Input: part model. Units: mm. Frame: model coordinates. Face numbers are marked on the shaded views. A direction names the side the tool comes from. Round coordinates to 2 decimals unless told otherwise and drop trailing zeros. Loops run counter-clockwise (first coordinate to the right, second up) from the corner with the lowest first, then second, coordinate; pieces in that order, holes last. Notation, with made-up numbers: M 1.25,31.25 L 36.25,31.25 A15 ccw 36.25,48.25 Z; hole C -37,59 d8. An arc over 180 degrees is marked long. Return JSON: item names as keys, results as strings. Group by question number.
1) Section C-C (z = 12). Output: boundary loops of the cut face in (x, y), plus the area to 3 significant figures.
2) Section B-B (x = 8.5). Output: boundary loops of the cut face in (y, z).
3) Material intervals for line 1 (Z direction, x = -2.5, y = 2); line 2 (Y direction, x = 7, z = 23); line 3 (Y direction, x = 3, z = -13.5), sorted ascending. Write a range as from..to.
4) Section D-D (x = -10.5). Output: boundary loops of the cut face in (y, z).
5) Section A-A (y = 2). Output: boundary loops of the cut face in (x, z).
6) Access query for the marked faces 1 and 2. Directions: +Z, -Z, +X, -X, +Y, -Y. A direction counts if a zero-diameter tool reaches every point of the face in a straight line with its end or side. Return the directions, or none.
7) Contact query for flat-ended pins moving along their axis: P1, Ø1, axis at x = 2, y = 2, coming from the -Z side; P2, Ø11, axis at x = 7, z = 25, coming from the +Y side; P3, Ø1.4, axis at y = 2.5, z = -17, coming from the -X side. Output: stop coordinate, or through.
from build123d import *

# Parameters (mm, degrees)
SKETCH_1_W          = 32.2
SKETCH_1_H          = 49.23
EXTRUDE_1_DEPTH     = 1.2
SKETCH_2_W          = 20.32
SKETCH_2_H          = 2
EXTRUDE_2_DEPTH     = 1.8
SKETCH_2_3_R        = 1.75
CUT_EXTRUDE_1_DEPTH = 1.8
EXTRUDE_3_DEPTH     = 1.46


with BuildPart() as part:
    # Sketch 1 → Extrude 1 (new body)
    with BuildSketch(Plane(origin=(0, 0, 0), x_dir=(1, 0, 0), z_dir=(0, 1, 0))):
        with Locations((0.963198928, -6.298805668)):
            Rectangle(SKETCH_1_W, SKETCH_1_H)
    extrude(amount=EXTRUDE_1_DEPTH)

    # Sketch 2 → Extrude 2 (add)
    with BuildSketch(Plane(origin=(0, 1.2, 0), x_dir=(1, 0, 0), z_dir=(0, 1, 0))):
        with Locations((0.963198928, 16.816194332)):
            Rectangle(SKETCH_2_W, SKETCH_2_H)
    extrude(amount=EXTRUDE_2_DEPTH)

    # Sketch 2_3 → Cut-Extrude 1 (cut)
    with BuildSketch(Plane(origin=(0, 1.2, 0), x_dir=(1, 0, 0), z_dir=(0, 1, 0))):
        with Locations(Location((15.063198928, -28.913805668, 0), (0, 0, 270))):
            Circle(SKETCH_2_3_R)
        with Locations(Location((15.063198928, 16.316194332, 0), (0, 0, 270))):
            Circle(SKETCH_2_3_R)
        with Locations(Location((-13.136801072, 16.316194332, 0), (0, 0, 270))):
            Circle(SKETCH_2_3_R)
        with Locations(Location((-13.136801072, -28.913805668, 0), (0, 0, 270))):
            Circle(SKETCH_2_3_R)
    extrude(amount=-CUT_EXTRUDE_1_DEPTH, mode=Mode.SUBTRACT)

    # Sketch 3 → Extrude 3 (add)
    with BuildSketch(Plane(origin=(0, 1.2, 0), x_dir=(1, 0, 0), z_dir=(0, 1, 0))):
        with BuildLine():
            Line((-9.986801072, 13.316194332), (11.913198928, 13.316194332))
            ThreePointArc((11.913198928, 13.316194332), (15.554798851, 11.807794255), (17.063198928, 8.166194332))
            Line((17.063198928, 8.166194332), (17.063198928, -20.763805668))
            ThreePointArc((17.063198928, -20.763805668), (15.554798851, -24.405405591), (11.913198928, -25.913805668))
            Line((11.913198928, -25.913805668), (-9.986801072, -25.913805668))
            ThreePointArc((-9.986801072, -25.913805668), (-13.628400995, -24.405405591), (-15.136801072, -20.763805668))
            Line((-15.136801072, -20.763805668), (-15.136801072, 8.166194332))
            ThreePointArc((-15.136801072, 8.166194332), (-13.628400995, 11.807794255), (-9.986801072, 13.316194332))
        make_face()
    extrude(amount=EXTRUDE_3_DEPTH)


solid = part.part
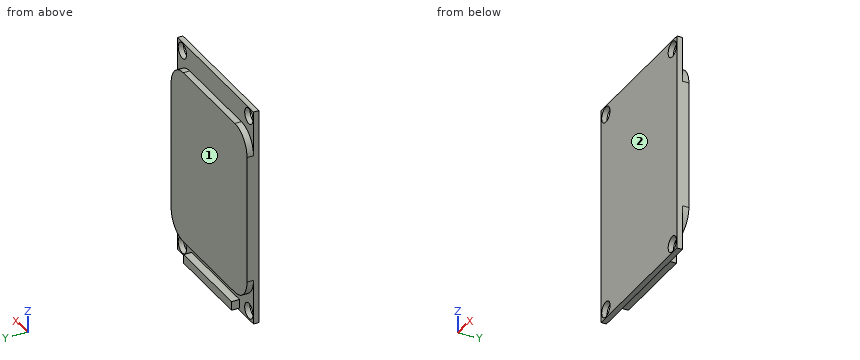
Returned:
{
 "1": {"outline": "M -15.14,0 L 17.06,0 L 17.06,2.66 L -15.14,2.66 Z", "area": "85.7 mm^2"},
 "2": {"outline": "M 0,-18.32 L 1.2,-18.32 L 1.2,-17.82 L 3,-17.82 L 3,-15.82 L 1.2,-15.82 L 1.2,-13.32 L 2.66,-13.32 L 2.66,25.91 L 1.2,25.91 L 1.2,30.91 L 0,30.91 Z"},
 "3": {"line 1": "z = -17.82..-15.82, -13.32..25.91", "line 2": "y = 0..2.66", "line 3": "y = 0..1.2"},
 "4": {"outline": "M 0,-18.32 L 1.2,-18.32 L 1.2,-13.29 L 2.66,-13.29 L 2.66,25.89 L 1.2,25.89 L 1.2,30.91 L 0,30.91 Z"},
 "5": {"outline": "M -15.14,-8.17 A5.15 ccw -9.99,-13.32 L 11.91,-13.32 A5.15 ccw 17.06,-8.17 L 17.06,20.76 A5.15 ccw 11.91,25.91 L -9.99,25.91 A5.15 ccw -15.14,20.76 Z; M -9.2,-17.82 L 11.12,-17.82 L 11.12,-15.82 L -9.2,-15.82 Z"},
 "6": {"face 1": "+Z, +X, -X, +Y", "face 2": "+Z, -Z, +X, -X, -Y"},
 "7": {"P1": "stops at z = -17.82", "P2": "stops at y = 2.66", "P3": "stops at x = -9.2"}
}
